```python
from build123d import *

# Parameters (mm, degrees)
SKETCH1_R           = 5
BOSS_EXTRUDE1_DEPTH = 4.1
FILLET1_R           = 0.6
CUT_EXTRUDE1_DEPTH  = 3.6
SKETCH3_R           = 3
BOSS_EXTRUDE2_DEPTH = 25


with BuildPart() as part:
    # Sketch1 → Boss-Extrude1 (new body)
    with BuildSketch(Plane(origin=(0, 0, 0), x_dir=(1, 0, 0), z_dir=(0, 1, 0))):
        with Locations(Location((0, 0, 0), (0, 0, 270))):
            Circle(SKETCH1_R)
    extrude(amount=BOSS_EXTRUDE1_DEPTH)

    # Fillet1
    fillet1_edges = [part.edges().sort_by_distance(p)[0] for p in [
        (0, 4.1, -5),
    ]]
    fillet(fillet1_edges, radius=FILLET1_R)

    # Sketch2 → Cut-Extrude1 (cut)
    with BuildSketch(Plane(origin=(0, 4.1, 0), x_dir=(1, 0, 0), z_dir=(0, 1, 0))):
        Polygon((0, -2.367136104), (2.05, -1.183568052), (2.05, 1.183568052), (0, 2.367136104), (-2.05, 1.183568052), (-2.05, -1.183568052), align=None)
    extrude(amount=-CUT_EXTRUDE1_DEPTH, mode=Mode.SUBTRACT)

    # Sketch3 → Boss-Extrude2 (add)
    with BuildSketch(Plane.XZ):
        with Locations(Location((0, 0, 0), (0, 0, 270))):
            Circle(SKETCH3_R)
    extrude(amount=BOSS_EXTRUDE2_DEPTH)


solid = part.part
```
Check sheet for the modelled part. Datum: model origin and axes. Units: mm. A direction names the side the tool comes from. Round coordinates to 2 decimals unless told otherwise and drop trailing zeros. Order: outer loops, then holes, each group sorted by start corner. A loop starts at its lowest first (then second) coordinate and runs counter-clockwise, first axis right, second up.
1) Section check B-B (y = -20). Record the boundary of the cut face in (x, z).
2) Mould release check, pull along X, two halves, no side actions. Record for faces 3 (the flat face through (-3.3, 0, -0.1)), 4 (the flat face through (-2.05, 2, 0)), 5 (the cylindrical face through (0.9, -12.32, -2.86)), 6 (the flat face through (1.039, 2.325, -1.767)): +X half, -X half, draft (parallel to the pull), parting line (faces both ways), or undercut.
3) Go/stop test with flat-tipped pins: pin 1 Ø1.5 at (y, z) = (-6, -3.5) entering from +X; pin 2 Ø1.5 at (x, z) = (-0.5, 0.5) entering from +Y; pin 3 Ø5 at (x, y) = (4, -0.5) entering from +Z. Record where each tip stops, or that it passes through.
4) Tool access check on faces 1 (the cylindrical face through (-4.88, 1.73, -1.08)), 2 (the flat face through (2.05, 2, 0)). Record the directions out of +Z, -Z, +X, -X, +Y, -Y that give a thin tool (end or side, any length) a straight path to the whole face; none if there is none.
5) Scan lines: line 1 (Y direction, x = -2, z = 3.75); line 2 (Y direction, x = -0.75, z = -0.5); line 3 (X direction, y = -20.5, z = 2.5). Record each from-to range of solid material in increasing order.
6) Section check A-A (z = 0). Record the boundary of the cut face in (x, y), and give its area (3 significant figures).
Result:
1. outline: circle Ø6 at (0, 0)
2. face 3: draft
2. face 4: undercut
2. face 5: parting line
2. face 6: undercut
3. pin 1: stops at x = 1.2
3. pin 2: stops at y = 0.5
3. pin 3: stops at z = 4.75
4. face 1: +Y, -Y
4. face 2: +Y
5. line 1: y = 0 to 4.1
5. line 2: y = -25 to 0.5
5. line 3: x = -1.66 to 1.66
6. outline: (-5, 0) - (-3, 0) - (-3, -25) - (3, -25) - (3, 0) - (5, 0) - (5, 3.5) arc R0.6 ccw to (4.4, 4.1) - (2.05, 4.1) - (2.05, 0.5) - (-2.05, 0.5) - (-2.05, 4.1) - (-4.4, 4.1) arc R0.6 ccw to (-5, 3.5) - close
6. area: 176 mm2
